from build123d import *

# Parameters (mm, degrees)
SKETCH1_W      = 148
SKETCH1_H      = 196
SKETCH1_R      = 13
EXTRUDE1_DEPTH = 36
SKETCH2_R      = 21.720880237
EXTRUDE2_DEPTH = 182.118745579
SKETCH3_R      = 16.5
EXTRUDE3_DEPTH = 6
SKETCH5_R      = 25
EXTRUDE5_DEPTH = 6
SKETCH4_R      = 7
EXTRUDE4_DEPTH = 182.118745579


# Read off the part's stored shape, not the designer's step: Cavity1
with BuildPart() as part:
    # Sketch1 → Extrude1 (new body)
    with BuildSketch(Plane.XY):
        with Locations((-74, 0)):
            Rectangle(SKETCH1_W, SKETCH1_H)
        with Locations((-120, 75)):
            Circle(SKETCH1_R, mode=Mode.SUBTRACT)
        with Locations((-120, -75)):
            Circle(SKETCH1_R, mode=Mode.SUBTRACT)
    extrude(amount=EXTRUDE1_DEPTH)

    # Cavity1 outline → Cavity1 (revolve, cut)
    with BuildSketch(Plane(origin=(-55, 0, 0), x_dir=(1, 0, 0), z_dir=(0, -1, 0))):
        with BuildLine():
            Line((32.16, 1.5075), (21.720880237, 1.5075))
            ThreePointArc((21.720880237, 1.5075), (19.980169175, 1.111079032), (18.582768743, 0))
            Line((18.582768743, 0), (32.16, 0))
            Line((32.16, 0), (32.16, 1.5075))
        make_face()
    revolve(axis=Axis((-55, 0, 0), (0, 0, 1)), mode=Mode.SUBTRACT)

    # Sketch2 → Extrude2 (cut, through all)
    with BuildSketch(Plane.XY):
        with Locations((-55, 0)):
            Circle(SKETCH2_R)
    extrude(amount=EXTRUDE2_DEPTH, mode=Mode.SUBTRACT)

    # Sketch3 → Extrude3 (cut)
    with BuildSketch(Plane.XY.offset(36)):
        with Locations((-120, 75)):
            Circle(SKETCH3_R)
        with Locations((-120, -75)):
            Circle(SKETCH3_R)
    extrude(amount=-EXTRUDE3_DEPTH, mode=Mode.SUBTRACT)

    # Sketch5 → Extrude5 (cut)
    with BuildSketch(Plane.XY.offset(36)):
        with Locations((-55, 0)):
            Circle(SKETCH5_R)
    extrude(amount=-EXTRUDE5_DEPTH, mode=Mode.SUBTRACT)

    # Sketch7 → Cut-Revolve2 (revolve, cut)
    with BuildSketch(Plane(origin=(0, 0, 0), x_dir=(1, 0, 0), z_dir=(0, 1, 0))):
        Polygon((-116.584356678, 3.471349293), (-103.64765553, -32.071944992), (-106.936579703, -33.269015494), (-102.122979844, -46.494272413), (-94.135592567, -43.587101195), (-111.885893574, 5.18145001), align=None)
    revolve(axis=Axis((-116.086721699, 0, -16.723130427), (0.34202014332566283, 0, 0.9396926207859105)), mode=Mode.SUBTRACT)

    # Mirror1: part across plane


with BuildPart() as part_1:
    add(part.part)
    add(part.part.mirror(Plane(origin=(0, 0, 0), x_dir=(0, 0, 1), z_dir=(1, 0, 0))))

    # Sketch4 → Extrude4 (cut, through all)
    with BuildSketch(Plane.XY.offset(36)):
        Circle(SKETCH4_R)
    extrude(amount=-EXTRUDE4_DEPTH, mode=Mode.SUBTRACT)

    # Sketch6 → Cut-Revolve1 (revolve, cut)
    with BuildSketch(Plane(origin=(0, 0, 0), x_dir=(-1, 0, 0), z_dir=(0, 0, -1))):
        with BuildLine():
            Line((-17.34, 2.5), (17.34, 2.5))
            ThreePointArc((17.34, 2.5), (19.107766953, 1.767766953), (19.84, 0))
            Line((19.84, 0), (-19.84, 0))
            ThreePointArc((-19.84, 0), (-19.107766953, 1.767766953), (-17.34, 2.5))
        make_face()
    revolve(axis=Axis((55, 0, 0), (-1, 0, 0)), mode=Mode.SUBTRACT)


solid = part_1.part
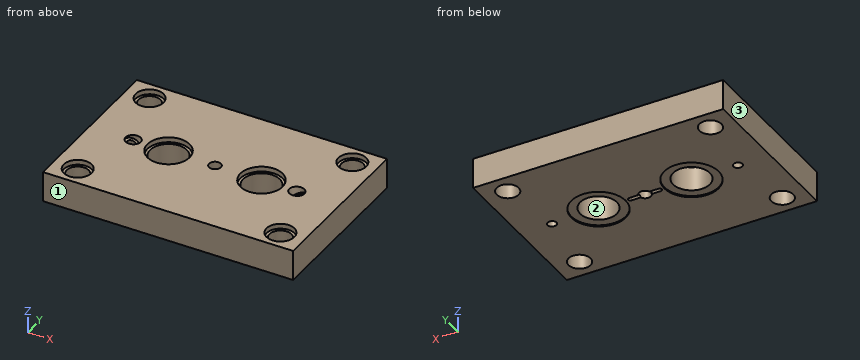
CAD build for the part. Positions are in the model's coordinates, mm. Face numbers are marked on the shaded views. Coordinates: 2 decimals unless noted, no trailing zeros. Order: outer loops, then holes, each group sorted by start corner. A loop starts at its lowest first (then second) coordinate and runs counter-clockwise, first axis right, second up.
Item 1: Band-saw the part on C-C on x = 55. List the corners of the cut face in (y, z), plus the area to 3 significant figures.
Check sheet entries:
outline: (-98, 0) - (-32.16, 0) - (-32.16, 1.51) - (-21.72, 1.51) - (-21.72, 30) - (-25, 30) - (-25, 36) - (-98, 36) - close; (21.72, 1.51) - (32.16, 1.51) - (32.16, 0) - (98, 0) - (98, 36) - (25, 36) - (25, 30) - (21.72, 30) - close
area: 5,420 mm2
Item 2: Pin check, flat tip, straight feed: pin 1 Ø16.5 at (x, y) = (116.5, -78.5) entering from +Z. Stop position of the tip, or through.
Check sheet entries:
pin 1: stops at z = 30
Item 3: Band-saw the part on D-D on z = 8. Give the number of separate pieces and of enclosed holes in the cut face, plus the area to 3 significant figures.
Check sheet entries:
separate pieces: 1
enclosed holes: 9
area: 52,600 mm2
Item 4: Band-saw the part on A-A on y = -75. List the corners of the cut face in (x, z).
Check sheet entries:
outline: (-148, 0) - (-133, 0) - (-133, 30) - (-136.5, 30) - (-136.5, 36) - (-148, 36) - close; (-107, 0) - (107, 0) - (107, 30) - (103.5, 30) - (103.5, 36) - (-103.5, 36) - (-103.5, 30) - (-107, 30) - close; (133, 0) - (148, 0) - (148, 36) - (136.5, 36) - (136.5, 30) - (133, 30) - close
Item 5: Drill centre lines: L1, parallel to X at y = 75, z = 12; L2, parallel to Y at x = -120, z = 19.5; L3, parallel to Y at x = -55, z = 10.5. Where is each one in solid material? Low to high.
Check sheet entries:
L1: x = -148 to -133, -107 to 107, 133 to 148
L2: y = -98 to -88, -62 to 62, 88 to 98
L3: y = -98 to -21.72, 21.72 to 98
Item 6: Two-plate mould, pull along X, no slides. Class the marked faces 1, 2 and 3: +X half, -X half, draft (parallel to the pull), parting line (faces both ways), or undercut.
Check sheet entries:
face 1: draft
face 2: undercut
face 3: -X half
Item 7: Band-saw the part on B-B on x = 120. List the corners of the cut face in (y, z).
Check sheet entries:
outline: (-98, 0) - (-88, 0) - (-88, 30) - (-91.5, 30) - (-91.5, 36) - (-98, 36) - close; (-62, 0) - (62, 0) - (62, 30) - (58.5, 30) - (58.5, 36) - (-58.5, 36) - (-58.5, 30) - (-62, 30) - close; (88, 0) - (98, 0) - (98, 36) - (91.5, 36) - (91.5, 30) - (88, 30) - close
